CAD build for the part. Positions are in the model's coordinates, mm. Coordinates: 2 decimals unless noted, no trailing zeros. Order: outer loops, then holes, each group sorted by start corner. A loop starts at its lowest first (then second) coordinate and runs counter-clockwise, first axis right, second up. Notation, with made-up numbers: M 61.25,70.25 L 74.25,70.25 A26 cw 74.25,97.25 Z; hole C -22.75,-29.5 d11. An arc over 180 degrees is marked long. Write item = value, one per line.
from build123d import *

# Parameters (mm, degrees)
SKETCH1_W           = 47.752
SKETCH1_H           = 63.5
SKETCH1_R           = 14.605
SKETCH1_R_2         = 2.794
BOSS_EXTRUDE1_DEPTH = 11.176
FILLET1_SIZE        = 5.08
CHAMFER1_SIZE       = 2.54


with BuildPart() as part:
    # Sketch1 → Boss-Extrude1 (new, symmetric)
    with BuildSketch(Plane(origin=(0, 0, 0), x_dir=(0, 0, -1), z_dir=(1, 0, 0))):
        Rectangle(SKETCH1_W, SKETCH1_H)
        Circle(SKETCH1_R, mode=Mode.SUBTRACT)
        with Locations((0, -25.4)):
            Circle(SKETCH1_R_2, mode=Mode.SUBTRACT)
        with Locations((0, 25.4)):
            Circle(SKETCH1_R_2, mode=Mode.SUBTRACT)
    extrude(amount=BOSS_EXTRUDE1_DEPTH, both=True)

    # Fillet1
    fillet1_edges = [part.edges().sort_by_distance(p)[0] for p in [
        (0, -31.75, -23.876),
        (0, -31.75, 23.876),
        (0, 31.75, 23.876),
        (0, 31.75, -23.876),
    ]]
    chamfer(fillet1_edges, length=FILLET1_SIZE)

    # Chamfer1
    # the kernel refuses this chamfer: 2.54 mm, written as the material it takes off along each edge
    with BuildSketch(Plane(origin=(-11.176, 0, 0), x_dir=(0, 0, -1), z_dir=(0, -1, 0))) as chamfer1_piece_1:
        Polygon((14.605 + CHAMFER1_SIZE, 0), (14.605, CHAMFER1_SIZE), (14.605, 0), align=None)
    revolve(axis=Axis((-11.176, 0, 0), (1, 0, 0)), mode=Mode.SUBTRACT)
    with BuildSketch(Plane(origin=(11.176, 0, 0), x_dir=(0, 0, -1), z_dir=(0, -1, 0))) as chamfer1_piece_2:
        Polygon((14.605 + CHAMFER1_SIZE, 0), (14.605, -CHAMFER1_SIZE), (14.605, 0), align=None)
    revolve(axis=Axis((11.176, 0, 0), (1, 0, 0)), mode=Mode.SUBTRACT)
    with BuildSketch(Plane(origin=(-11.176, -25.4, 0), x_dir=(0, 0, -1), z_dir=(0, -1, 0))) as chamfer1_piece_3:
        Polygon((2.794 + CHAMFER1_SIZE, 0), (2.794, CHAMFER1_SIZE), (2.794, 0), align=None)
    revolve(axis=Axis((-11.176, -25.4, 0), (1, 0, 0)), mode=Mode.SUBTRACT)
    with BuildSketch(Plane(origin=(11.176, -25.4, 0), x_dir=(0, 0, -1), z_dir=(0, -1, 0))) as chamfer1_piece_4:
        Polygon((2.794 + CHAMFER1_SIZE, 0), (2.794, -CHAMFER1_SIZE), (2.794, 0), align=None)
    revolve(axis=Axis((11.176, -25.4, 0), (1, 0, 0)), mode=Mode.SUBTRACT)
    with BuildSketch(Plane(origin=(-11.176, 25.4, 0), x_dir=(0, 0, -1), z_dir=(0, -1, 0))) as chamfer1_piece_5:
        Polygon((2.794 + CHAMFER1_SIZE, 0), (2.794, CHAMFER1_SIZE), (2.794, 0), align=None)
    revolve(axis=Axis((-11.176, 25.4, 0), (1, 0, 0)), mode=Mode.SUBTRACT)
    with BuildSketch(Plane(origin=(11.176, 25.4, 0), x_dir=(0, 0, -1), z_dir=(0, -1, 0))) as chamfer1_piece_6:
        Polygon((2.794 + CHAMFER1_SIZE, 0), (2.794, -CHAMFER1_SIZE), (2.794, 0), align=None)
    revolve(axis=Axis((11.176, 25.4, 0), (1, 0, 0)), mode=Mode.SUBTRACT)
    with BuildSketch(Plane(origin=(-11.176, 31.75, -25.328074789), x_dir=(-0.02749587661058663, -0.9996219169112968, 0), z_dir=(0, 0, 1)), Plane(origin=(11.176, -31.75, 25.328074789), x_dir=(-0.9996219169112968, -0.02749587661058591, 0), z_dir=(0, 0, -1))) as chamfer1_piece_7:
        Polygon((CHAMFER1_SIZE * 0.999621916911, CHAMFER1_SIZE * 0.0274958766106), (-CHAMFER1_SIZE * 0.0274958766106, CHAMFER1_SIZE * 0.999621916911), (0, 0), align=None)
    extrude(amount=50.656149579, mode=Mode.SUBTRACT)
    with BuildSketch(Plane(origin=(11.176, 31.75, -25.328074789), x_dir=(0.02749587661058663, -0.9996219169112968, 0), z_dir=(0, 0, 1)), Plane(origin=(-11.176, -31.75, 25.328074789), x_dir=(0.9996219169112968, -0.02749587661058591, 0), z_dir=(0, 0, -1))) as chamfer1_piece_8:
        Polygon((CHAMFER1_SIZE * 0.999621916911, -CHAMFER1_SIZE * 0.0274958766106), (-CHAMFER1_SIZE * 0.0274958766106, -CHAMFER1_SIZE * 0.999621916911), (0, 0), align=None)
    extrude(amount=50.656149579, mode=Mode.SUBTRACT)
    with BuildSketch(Plane(origin=(-11.176, -33.202074789, -23.876), x_dir=(-0.02749587661058663, 0, 0.9996219169112968), z_dir=(0, 1, 0)), Plane(origin=(-11.176, 33.202074789, 23.876), x_dir=(-0.02749587661058663, 0, -0.9996219169112968), z_dir=(0, -1, 0))) as chamfer1_piece_9:
        Polygon((CHAMFER1_SIZE * 0.999621916911, CHAMFER1_SIZE * 0.0274958766106), (-CHAMFER1_SIZE * 0.0274958766106, CHAMFER1_SIZE * 0.999621916911), (0, 0), align=None)
    extrude(amount=66.404149579, mode=Mode.SUBTRACT)
    with BuildSketch(Plane(origin=(-11.176, -36.368874379, -14.177125621), x_dir=(-0.027495876610586566, 0.7068394360706737, 0.7068394360706733), z_dir=(0, 0.7071067811865474, -0.7071067811865477)), Plane(origin=(11.176, -36.368874379, -14.177125621), x_dir=(-0.9996219169112966, -0.019442520806015103, -0.019442520806015093), z_dir=(0, 0.7071067811865474, -0.7071067811865477)), Plane(origin=(11.176, 22.051125621, 28.494874379), x_dir=(0.027495876610586632, -0.7068394360706737, -0.7068394360706733), z_dir=(0, 0.7071067811865474, -0.7071067811865477)), Plane(origin=(11.176, 36.368874379, -14.177125621), x_dir=(0.027495876610586566, -0.7068394360706737, 0.7068394360706733), z_dir=(0, -0.7071067811865474, -0.7071067811865477))) as chamfer1_piece_10:
        Polygon((CHAMFER1_SIZE * 0.999621916911, CHAMFER1_SIZE * 0.0274958766106), (-CHAMFER1_SIZE * 0.0274958766106, CHAMFER1_SIZE * 0.999621916911), (0, 0), align=None)
    extrude(amount=20.248354476, mode=Mode.SUBTRACT)
    with BuildSketch(Plane(origin=(-11.176, -36.368874379, 14.177125621), x_dir=(-0.027495876610586566, 0.7068394360706737, -0.7068394360706733), z_dir=(0, 0.7071067811865474, 0.7071067811865477)), Plane(origin=(-11.176, 22.051125621, 28.494874379), x_dir=(-0.027495876610586632, -0.7068394360706737, -0.7068394360706733), z_dir=(0, 0.7071067811865474, -0.7071067811865477)), Plane(origin=(-11.176, 36.368874379, -14.177125621), x_dir=(-0.027495876610586566, -0.7068394360706737, 0.7068394360706733), z_dir=(0, -0.7071067811865474, -0.7071067811865477)), Plane(origin=(11.176, -36.368874379, 14.177125621), x_dir=(-0.9996219169112966, -0.019442520806015457, 0.019442520806015447), z_dir=(0, 0.7071067811865474, 0.7071067811865477))) as chamfer1_piece_11:
        Polygon((CHAMFER1_SIZE * 0.999621916911, -CHAMFER1_SIZE * 0.0274958766106), (-CHAMFER1_SIZE * 0.0274958766106, -CHAMFER1_SIZE * 0.999621916911), (0, 0), align=None)
    extrude(amount=20.248354476, mode=Mode.SUBTRACT)
    with BuildSketch(Plane(origin=(11.176, -33.202074789, -23.876), x_dir=(0.02749587661058663, 0, 0.9996219169112968), z_dir=(0, 1, 0)), Plane(origin=(11.176, 33.202074789, 23.876), x_dir=(0.02749587661058663, 0, -0.9996219169112968), z_dir=(0, -1, 0))) as chamfer1_piece_12:
        Polygon((CHAMFER1_SIZE * 0.999621916911, -CHAMFER1_SIZE * 0.0274958766106), (-CHAMFER1_SIZE * 0.0274958766106, -CHAMFER1_SIZE * 0.999621916911), (0, 0), align=None)
    extrude(amount=66.404149579, mode=Mode.SUBTRACT)


solid = part.part
(1) Slice it at B-B, the plane x = 0. Write the cut outline in (y, z) (3 decimals), then the cut area to 3 significant figures.
Evaluation:
outline = M -31.75,-18.796 L -26.67,-23.876 L 26.67,-23.876 L 31.75,-18.796 L 31.75,18.796 L 26.67,23.876 L -26.67,23.876 L -31.75,18.796 Z; hole C -25.4,0 d5.588; hole C 0,0 d29.21; hole C 25.4,0 d5.588
area = 2,260 mm²
(2) Pin check, flat tips, straight feed: pin 1 Ø8 at (y, z) = (7, -7) entering from -X; pin 2 Ø6.5 at (y, z) = (-25.4, 0) entering from -X. Stop position of each tip, or through.
Evaluation:
pin_1 = through
pin_2 = -9.09
(3) Wall check: line 1 (Y direction, x = 1.25, z = 0) (3 decimals); line 2 (Y direction, x = 3.5, z = 3.5); line 3 (Y direction, x = 8, z = -13). Give the ranges that are in metal, low to high. Write a range as from..to.
Evaluation:
line_1 = -31.75..-28.194, -22.606..-14.605, 14.605..22.606, 28.194..31.75
line_2 = -31.75..-14.18, 14.18..31.75
line_3 = -31.75..-6.66, 6.66..31.75
(4) Slice it at C-C, the plane z = 0. Write the cut outline in (x, y) (3 decimals), then the cut area to 3 significant figures.
Evaluation:
outline = M -11.176,-20.066 L -8.636,-22.606 L 8.636,-22.606 L 11.176,-20.066 L 11.176,-17.145 L 8.636,-14.605 L -8.636,-14.605 L -11.176,-17.145 Z; M -11.176,17.145 L -8.636,14.605 L 8.636,14.605 L 11.176,17.145 L 11.176,20.066 L 8.636,22.606 L -8.636,22.606 L -11.176,20.066 Z; M -10.414,-29.972 L -8.636,-31.75 L 8.636,-31.75 L 10.414,-29.972 L 8.636,-28.194 L -8.636,-28.194 Z; M -10.414,29.972 L -8.636,28.194 L 8.636,28.194 L 10.414,29.972 L 8.636,31.75 L -8.636,31.75 Z
area = 467 mm²
(5) Pull direction Y, two halves, no side cores. Call faces 1 (the face through (-0.121, -28.128, 0.606)), 2 (the face through (9.92, -0.37, -22.59)), 3 (the face through (9.924, 30.462, -0.263)): +Y half, -Y half, draft (parallel to the pull), parting line (faces both ways), or undercut.
Evaluation:
face_1 = undercut
face_2 = draft
face_3 = +Y half
(6) Slice it at A-A, the plane y = 0. Write the cut outline in (x, z) (3 decimals), then the cut area to 3 significant figures.
Evaluation:
outline = M -11.176,-21.336 L -8.636,-23.876 L 8.636,-23.876 L 11.176,-21.336 L 11.176,-17.145 L 8.636,-14.605 L -8.636,-14.605 L -11.176,-17.145 Z; M -11.176,17.145 L -8.636,14.605 L 8.636,14.605 L 11.176,17.145 L 11.176,21.336 L 8.636,23.876 L -8.636,23.876 L -11.176,21.336 Z
area = 389 mm²
